Autodesk Inventor part; units mm, degrees
ref_plane "YZ Plane" through (0, 0, 0) normal (1, 0, 0) x (0, 1, 0)
ref_plane "XZ Plane" through (0, 0, 0) normal (0, 1, 0) x (-1, 0, 0)
ref_plane "XY Plane" through (0, 0, 0) normal (0, 0, 1) x (1, 0, 0)
sketch "スケッチ1" plane through (0, 0, 0) normal (0, 1, 0) x (-1, 0, 0)
  line L0 (0, 0) -> (106, 0)
  line L1 (106, 0) -> (106, -113)
  line L2 (106, -113) -> (0, -113)
  line L3 (0, -113) -> (0, 0)
  dimension "d0" = 106
  dimension "d1" = 113
extrude "押し出し1" add sketch "スケッチ1" along normal blind 3
sketch "スケッチ3" plane through (0, 3, 0) normal (0, 1, 0) x (1, 0, 0)
  line L0 (-106, 113) -> (-106, 0)
  line L1 (0, 113) -> (-106, 113)
  circle A0 centre (-53, 60) radius 35.5
  line L2 (-106, 0) -> (0, 0)
  line L3 (-106, 60) -> (0, 60)
  line L4 (0, 0) -> (0, 113)
  circle A1 centre (-53, 60) radius 53
  point P0 (-53, 113)
  point P1 (0, 60)
  point P2 (-106, 60)
  dimension "d17" = 71
  dimension "d49" = 53
  dimension "d50" = 0
  dimension "d52" = 106
extrude "押し出し2" cut sketch "スケッチ3" against normal blind 3 contours L1 A1 L0 | L1 L4 A1 | L3 A0 | A0 L3
sketch "スケッチ4" plane through (0, 3, 0) normal (0, 1, 0) x (1, 0, 0)
  line L0 (-106, 113) -> (-106, 0)
  line L1 (-106, 5) -> (0, 5)
  line L2 (0, 0) -> (0, 113)
  line L3 (-106, 0) -> (0, 0)
  line L4 (0, 113) -> (-106, 113)
  line L5 (-106, 0) -> (0, 0)
  line L6 (-101, 0) -> (-101, 113)
  line L7 (-5, 113) -> (-5, 0)
  point P0 (-101, 5)
  point P1 (-5, 5)
  dimension "d22" = 5
  dimension "d24" = 5
  dimension "d25" = 5
hole "穴2" at (-101, 3, -5) at (-5, 3, -5) direction (0, -1, 0) diameter 3.2 end through all
sketch "スケッチ5" plane through (0, 3, 0) normal (0, 1, 0) x (1, 0, 0)
  line L0 (-106, 113) -> (-106, 0)
  line L1 (-106, 60) -> (0, 60)
  circle A0 centre (-53, 60) radius 49
  line L2 (0, 113) -> (-106, 113)
  line L3 (-53, 60) -> (-7.7299, 78.7515)
  point P0 (0, 0)
  point P1 (-34.2485, 105.2701)
  point P2 (-71.7515, 105.2701)
  point P3 (-98.2701, 78.7515)
  point P4 (-98.2701, 41.2485)
  point P5 (-71.7515, 14.7299)
  point P6 (-34.2485, 14.7299)
  point P7 (-7.7299, 41.2485)
  dimension "d35" = 98
  dimension "d36" = 53
  dimension "d37" = 22.5
  dimension "d40" = 360
hole "穴3" at (-7.7299, 3, -78.7515) at (-34.2485, 3, -105.2701) at (-71.7515, 3, -105.2701) at (-98.2701, 3, -78.7515) at (-98.2701, 3, -41.2485) at (-71.7515, 3, -14.7299) at (-34.2485, 3, -14.7299) at (-7.7299, 3, -41.2485) direction (0, -1, 0) diameter 4.2 end through all
equation "\"d47\" = Thickness"
equation "\"BendRadius\" = Thickness"
equation "\"BendReliefWidth\" = Thickness"
equation "\"BendReliefDepth\" = 0.5 * Thickness"
equation "\"CornerReliefSize\" = 4 * Thickness"
equation "\"MinimumRemnant\" = 2 * Thickness"
equation "\"TransitionRadius\" = BendRadius"
equation "\"JacobiRadiusSize\" = BendRadius"
equation "\"GapSize\" = Thickness"
properties part number "link2_plate1" material "アルミニウム 6061"
Part model, mm, in its own coordinate system. Give positions to 0.01 mm unless a question says otherwise; leave off trailing zeros. Write each loop counter-clockwise with the first axis right and the second up, starting at its lowest first coordinate (ties: lowest second). Pieces come first, ordered by that corner, then holes.
1) Cut at B-B on y = 1.05. State how many separate pieces and enclosed holes the cut face has, then the cut area to 3 significant figures.
Resolved:
separate pieces: 1
enclosed holes: 11
area: 6,690 mm2
2) Probe L1, parallel to Z at x = -53, y = 0.8; L2, parallel to X at y = 0.8, z = -5; L3, parallel to Z at x = -45, y = 2.65. List the from-to ranges inside material, lowest first.
Resolved:
L1: z = -113 to -95.5, -24.5 to 0
L2: x = -106 to -102.6, -99.4 to -6.6, -3.4 to 0
L3: z = -112.39 to -94.59, -25.41 to 0
3) Cut at C-C on z = -70.5. Write the cut outline in (x, y).
Resolved:
outline: (-104.95, 0) - (-86.91, 0) - (-86.91, 3) - (-104.95, 3) - close; (-19.09, 0) - (-1.05, 0) - (-1.05, 3) - (-19.09, 3) - close
4) Two-plate mould, pull along Z, no slides. Class faces 1 (the face through (-4.03, 1.48, -6.27)), 2 (the face through (-51.835, 1.521, -112.987)), 3 (the face through (-36.33, 1.48, -105.54)), 4 (the face through (-29, 3, -31)): released by +Z, released by -Z, zero draft, split by the parting line, or undercut.
Resolved:
face 1: undercut
face 2: released by -Z
face 3: undercut
face 4: zero draft
5) Cut at A-A on x = -53. Write the cut outline in (y, z).
Resolved:
outline: (0, -113) - (3, -113) - (3, -95.5) - (0, -95.5) - close; (0, -24.5) - (3, -24.5) - (3, 0) - (0, 0) - close
6) Cut at D-D on x = -15. Write the cut outline in (y, z).
Resolved:
outline: (0, -96.95) - (3, -96.95) - (3, 0) - (0, 0) - close
